```python
from build123d import *


with BuildPart() as part:
    # Эскиз2 → Повернуть1 (revolve)
    with BuildSketch(Plane.XY, mode=Mode.PRIVATE) as revolve_1_sk:
        with BuildLine():
            Line((99.47989222, 92.177858052), (27.175004903, 23.67849112))
            ThreePointArc((27.175004903, 23.67849112), (27.112626839, 23.538704015), (27.167363296, 23.395751653))
            Line((27.167363296, 23.395751653), (27.236137761, 23.323156385))
            ThreePointArc((27.236137761, 23.323156385), (27.375924866, 23.260778321), (27.518877227, 23.315514778))
            Line((27.518877227, 23.315514778), (99.823764544, 91.81488171))
            ThreePointArc((99.823764544, 91.81488171), (99.886142609, 91.954668814), (99.831406152, 92.097621176))
            Line((99.831406152, 92.097621176), (99.762631687, 92.170216445))
            ThreePointArc((99.762631687, 92.170216445), (99.622844582, 92.232594509), (99.47989222, 92.177858052))
        make_face()
    revolve(revolve_1_sk.sketch.rotate(Axis((0, -32.617744242, 0), (0, 1, 0)), 90), axis=Axis((0, -32.617744242, 0), (0, 1, 0)))


solid = part.part
```
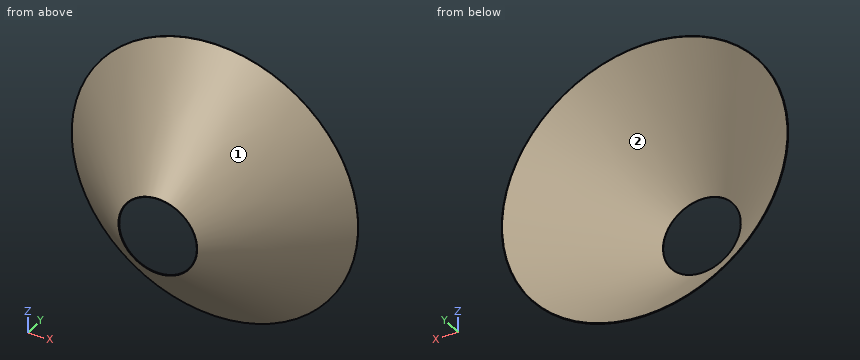
Could you check a few things on this model? Use its own coordinates, in mm. Face numbers are marked on the shaded views. Give positions to 0.01 mm unless a question says otherwise; leave off trailing zeros. Order: outer loops, then holes, each group sorted by start corner. A loop starts at its lowest first (then second) coordinate and runs counter-clockwise, first axis right, second up.
Q1. We'd pull the mould along Z, two halves only. Please class the marked faces 1 and 2: +Z half, -Z half, draft (parallel to the pull), parting line (faces both ways), or undercut.
Q2. Suppose I cut it at C-C, the plane y = 50.5. Write out the boundary of the cut face in (x, z), and give its area (3 significant figures).
Q3. I'm going to push flat-ended pins straight in: P1, Ø5, axis at x = -28, z = -54, coming from the -Y side; P2, Ø1.5, axis at x = 71, z = 56.5, coming from the -Y side; P3, Ø1, axis at y = 52.5, z = 7.5, coming from the -X side. Where does each tip first touch, or does it pass through?
Q4. Suppose I cut it at D-D, the plane y = 85. Write out the boundary of the cut face in (x, z).
Q5. If I drill on line 1 along X through (y, z) = (53, -35); line 2 along X through (y, z) = (29, -8); line 3 along Z through (x, y) = (33.5, 67), over which ranges is the centre line in solid material (lowest first)?
Solution:
1. face 1: parting line
1. face 2: undercut
2. outline: circle Ø112.43 at (0, 0); hole circle Ø110.97 at (0, 0)
2. area: 255 mm2
3. P1: stops at y = 52.5
3. P2: stops at y = 82.5
3. P3: stops at x = -58.38
4. outline: circle Ø185.26 at (0, 0); hole circle Ø183.81 at (0, 0)
5. line 1: x = -47.31 to -46.41, 46.41 to 47.31
5. line 2: x = -32.55 to -31.8, 31.8 to 32.55
5. line 3: z = -65.57 to -64.75, 64.75 to 65.57
